Input: part model. Units: mm. Frame: model coordinates. Give positions to 0.01 mm unless a question says otherwise; leave off trailing zeros. Order: outer loops, then holes, each group sorted by start corner. A loop starts at its lowest first (then second) coordinate and runs counter-clockwise, first axis right, second up.
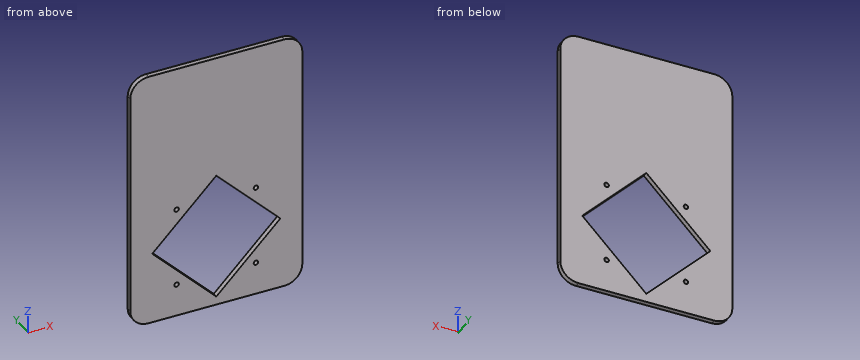
Autodesk Inventor part; units mm, degrees
ref_plane "YZ Plane" through (0, 0, 0) normal (1, 0, 0) x (0, 1, 0)
ref_plane "XZ Plane" through (0, 0, 0) normal (0, 1, 0) x (-1, 0, 0)
ref_plane "XY Plane" through (0, 0, 0) normal (0, 0, 1) x (1, 0, 0)
sketch "Sketch1" plane through (0, 0, 0) normal (0, 1, 0) x (-1, 0, 0)
  line L0 (-47.5, 72) -> (47.5, 72)
  line L1 (47.5, 72) -> (47.5, -72)
  line L2 (47.5, -72) -> (-47.5, -72)
  line L3 (-47.5, -72) -> (-47.5, 72)
  line L4 (-47.5, 72) -> (47.5, -72) construction
  line L5 (47.5, 72) -> (-47.5, -72) construction
  line L6 (0, 3.3553) -> (35.3553, -32)
  line L7 (35.3553, -32) -> (0, -67.3553)
  line L8 (0, -67.3553) -> (-35.3553, -32)
  line L9 (-35.3553, -32) -> (0, 3.3553)
  line L10 (0, 3.3553) -> (0, -67.3553) construction
  line L11 (35.3553, -32) -> (-35.3553, -32) construction
  point P0 (0, 0)
  point P1 (0, -32)
  point P2 (0, -32)
  point P3 (0, 0)
  dimension "d0" = 95
  dimension "d1" = 144
  dimension "d2" = 50
  dimension "d3" = 40
extrude "Extrusion1" add sketch "Sketch1" along normal blind 2.8
sketch "Sketch2" plane through (0, 2.8, 0) normal (0, 1, 0) x (1, 0, 0)
  line L0 (-35.3553, 32) -> (0, 67.3553) construction
  line L1 (0, 67.3553) -> (35.3553, 32) construction
  line L2 (35.3553, 32) -> (0, -3.3553) construction
  line L3 (0, -3.3553) -> (-35.3553, 32) construction
  line L4 (0, 75.8406) -> (-43.8406, 32)
  line L5 (-43.8406, 32) -> (0, -11.8406)
  line L6 (0, -11.8406) -> (43.8406, 32)
  line L7 (43.8406, 32) -> (0, 75.8406)
  point P0 (0, 0)
  point P1 (-21.9203, 53.9203)
  point P2 (21.9203, 53.9203)
  point P3 (21.9203, 10.0797)
  point P4 (-21.9203, 10.0797)
  dimension "d6" = 6
hole "Hole1" at (-21.9203, 2.8, -53.9203) at (21.9203, 2.8, -53.9203) at (21.9203, 2.8, -10.0797) at (-21.9203, 2.8, -10.0797) direction (0, -1, 0) diameter 2.5 end through all
fillet "Fillet1" radius 10 4 edges at (-47.5, 1.4, 72) (47.5, 1.4, 72) (47.5, 1.4, -72) (-47.5, 1.4, -72)
1) Cut plane A-A (x = -17). Return the cut outline in (y, z), then the cut area to 3 significant figures.
2) Line query: probe 1 along Z at (x, y) = (-18, 2.5); probe 2 along Z at (x, y) = (-34, 1.3); probe 3 along X at (y, z) = (0.75, -27). Output: solid intervals per line, ascending.
3) Cut plane B-B (z = 1.5). Return the cut outline in (x, y).
4) Cut plane C-C (y = 2.15). Return the cut outline in (x, z), then the cut area to 3 significant figures.
Geometry says:
1. outline: (0, -72) - (2.8, -72) - (2.8, -50.36) - (0, -50.36) - close; (0, -13.64) - (2.8, -13.64) - (2.8, 72) - (0, 72) - close
1. area: 300 mm2
2. probe 1: z = -72 to -49.36, -14.64 to 72
2. probe 2: z = -72 to -33.36, -30.64 to 72
2. probe 3: x = -47.5 to -30.36, 30.36 to 47.5
3. outline: (-47.5, 0) - (-1.86, 0) - (-1.86, 2.8) - (-47.5, 2.8) - close; (1.86, 0) - (47.5, 0) - (47.5, 2.8) - (1.86, 2.8) - close
4. outline: (-47.5, -62) arc R10 ccw to (-37.5, -72) - (37.5, -72) arc R10 ccw to (47.5, -62) - (47.5, 62) arc R10 ccw to (37.5, 72) - (-37.5, 72) arc R10 ccw to (-47.5, 62) - close; hole (-35.36, -32) - (0, -67.36) - (35.36, -32) - (0, 3.36) - close; hole circle Ø2.5 at (-21.92, -53.92); hole circle Ø2.5 at (-21.92, -10.08); hole circle Ø2.5 at (21.92, -53.92); hole circle Ø2.5 at (21.92, -10.08)
4. area: 11,100 mm2
